Geometry: see drawing. Coordinates: mm, zero at the bounding-box minimum. Give positions to 0.01 mm unless a question says otherwise; leave off trailing zeros. Write each loop counter-clockwise with the first axis right and the second up, starting at its lowest first coordinate (ties: lowest second). Pieces come first, ordered by that corner, then holes. Notation, with made-up numbers: (64.5, 50.25) - (114.5, 50.25) arc R25 cw to (114.5, 86.25) - close; hole circle Ø10 at (36.5, 56.25). An arc over 180 degrees is marked (long way). Use a Markdown table: item, result. Add a question column.
1. Material intervals for probe 1 along X at (y, z) = (4, 79.65); probe 2 along X at (y, z) = (4.5, 96); probe 3 along X at (y, z) = (5.25, 21.95), sorted ascending.
2. Section query A-A, the plane z = 79.65. Return loops of the section in (x, y), plus the area to 3 significant figures.
3. Section query C-C, the plane y = 2.75. Count the separate pieces of the cut face and the enclosed holes in it, plus the area to 3 significant figures.
4. Section query B-B, the plane z = 21.95. Return loops of the section in (x, y), plus the area to 3 significant figures.
5. Section query D-D, the plane x = 68.5. Return loops of the section in (y, z), plus the area to 3 significant figures.
6. Pin query (flat end, axial travel): pin 1 (1.5 mm diameter, centred on y = 3.5, z = 54, fed in from +X); pin 2 (1.9 mm diameter, centred on x = 17, y = 2.5, fed in from +Z); pin 3 (2 mm diameter, centred on x = 23, y = 5.5, fed in from -Z). Return the tip coordinate at first contact, or that it passes through.
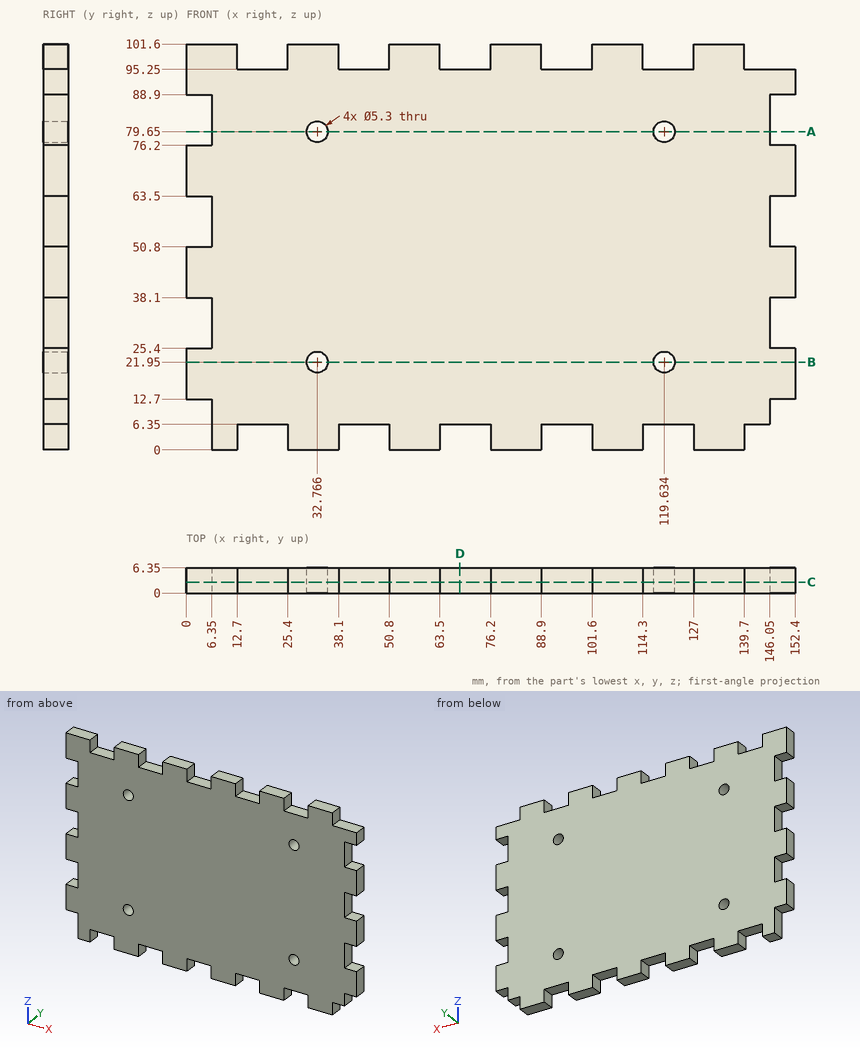
Result sheet:
| question | item | result |
|---|---|---|
| 1 | probe 1 | x = 6.35 to 30.12, 35.42 to 116.98, 122.28 to 146.05 |
| 1 | probe 2 | x = 0 to 12.7, 25.4 to 38.1, 50.8 to 63.5, 76.2 to 88.9, 101.6 to 114.3, 127 to 139.7 |
| 1 | probe 3 | x = 0 to 30.12, 35.42 to 116.98, 122.28 to 152.4 |
| 2 | outline | (6.35, 0) - (30.12, 0) - (30.12, 6.35) - (6.35, 6.35) - close; (35.42, 0) - (116.98, 0) - (116.98, 6.35) - (35.42, 6.35) - close; (122.28, 0) - (146.05, 0) - (146.05, 6.35) - (122.28, 6.35) - close |
| 2 | area | 820 mm² |
| 3 | separate pieces | 1 |
| 3 | enclosed holes | 4 |
| 3 | area | 13,800 mm² |
| 4 | outline | (0, 0) - (30.12, 0) - (30.12, 6.35) - (0, 6.35) - close; (35.42, 0) - (116.98, 0) - (116.98, 6.35) - (35.42, 6.35) - close; (122.28, 0) - (152.4, 0) - (152.4, 6.35) - (122.28, 6.35) - close |
| 4 | area | 900 mm² |
| 5 | outline | (0, 6.35) - (6.35, 6.35) - (6.35, 95.25) - (0, 95.25) - close |
| 5 | area | 565 mm² |
| 6 | pin 1 | stops at x = 146.05 |
| 6 | pin 2 | stops at z = 95.25 |
| 6 | pin 3 | stops at z = 6.35 |
